The model under review builds one solid part; all positions refer to its coordinate system, in mm. A direction names the side the tool comes from. Round coordinates to 2 decimals unless told otherwise and drop trailing zeros. Write each loop counter-clockwise with the first axis right and the second up, starting at its lowest first coordinate (ties: lowest second). Pieces come first, ordered by that corner, then holes. Notation, with made-up numbers: (-39, 37) -> (-32, 37) arc R6 cw to (-32, 43) -> close; hole circle Ø4 at (-5.5, -39.75). An arc over 180 degrees is marked (long way). Use CSV: the item, a comma, the result in double quotes. Start each with the question number.
1) Take a section at B-B, the plane x = -46.5. Give the boundary of the cut face in (y, z).
2) Mouldability with a two-part tool opening along Z and no side actions: class faces 5 (the face through (4.75, 1, 52)), 6 (the face through (-40, 2, -54)), 7 (the face through (-52, 1, -4.75)) as released by +Z, released by -Z, zero draft, split by the parting line, or undercut.
3) Take a section at A-A, the plane z = 6.5. Give the boundary of the cut face in (x, y).
4) For pin 1 Ø1.5 at (y, z) = (2, -26) entering from -X; pin 2 Ø1.5 at (x, y) = (-52, 1) entering from +Z; pin 3 Ø1.5 at (y, z) = (1.5, -52) entering from -X, all flat-tipped, find the tip position at first contact; note any pin that passes through.
5) Wall thickness on probe 1 along X at (y, z) = (2.3, 48): over which ranges is the line inside the solid? List them lowest first. Write a range as [from, to].
6) Machinability: for faces 1 (the face through (50, 1, 47)), 2 (the face through (50, 1, -47)), 3 (the face through (-52, 1, -44.75)), 4 (the face through (52, 1, 4.75)), which of the approach directions +Z, -Z, +X, -X, +Y, -Y give a long, thin tool a straight path to every point of the face, cutting with its end or side? Answer none if there is none.
from build123d import *

# Parameters (mm, degrees)
SKETCH2_W           = 100
SKETCH2_H           = 100
BOSS_EXTRUDE1_DEPTH = 3
SKETCH4_W           = 9.5
SKETCH4_H           = 3
BOSS_EXTRUDE2_DEPTH = 4
SKETCH5_W           = 9.5
SKETCH5_H           = 3
BOSS_EXTRUDE3_DEPTH = 4
SKETCH6_W           = 9.5
SKETCH6_H           = 3
BOSS_EXTRUDE4_DEPTH = 4
SKETCH7_W           = 9.5
SKETCH7_H           = 3
BOSS_EXTRUDE5_DEPTH = 4


with BuildPart() as part:
    # Sketch2 → Boss-Extrude1 (new body)
    with BuildSketch(Plane(origin=(0, 0, 0), x_dir=(1, 0, 0), z_dir=(0, 1, 0))):
        Rectangle(SKETCH2_W, SKETCH2_H)
    extrude(amount=BOSS_EXTRUDE1_DEPTH)

    # Sketch4 → Boss-Extrude2 (add)
    with BuildSketch(Plane.XY.offset(50)):
        with Locations((-40, 1.5)):
            Rectangle(SKETCH4_W, SKETCH4_H)
        with Locations((-20, 1.5)):
            Rectangle(SKETCH4_W, SKETCH4_H)
        with Locations((0, 1.5)):
            Rectangle(SKETCH4_W, SKETCH4_H)
        with Locations((20, 1.5)):
            Rectangle(SKETCH4_W, SKETCH4_H)
        with Locations((40, 1.5)):
            Rectangle(SKETCH4_W, SKETCH4_H)
    extrude(amount=BOSS_EXTRUDE2_DEPTH)

    # Sketch5 → Boss-Extrude3 (add)
    with BuildSketch(Plane.ZY.offset(50)):
        with Locations((-40, 1.5)):
            Rectangle(SKETCH5_W, SKETCH5_H)
        with Locations((-20, 1.5)):
            Rectangle(SKETCH5_W, SKETCH5_H)
        with Locations((0, 1.5)):
            Rectangle(SKETCH5_W, SKETCH5_H)
        with Locations((20, 1.5)):
            Rectangle(SKETCH5_W, SKETCH5_H)
        with Locations((40, 1.5)):
            Rectangle(SKETCH5_W, SKETCH5_H)
    extrude(amount=BOSS_EXTRUDE3_DEPTH)

    # Sketch6 → Boss-Extrude4 (add)
    with BuildSketch(Plane(origin=(50, 0, 0), x_dir=(0, 0, -1), z_dir=(1, 0, 0))):
        with Locations((-40, 1.5)):
            Rectangle(SKETCH6_W, SKETCH6_H)
        with Locations((-20, 1.5)):
            Rectangle(SKETCH6_W, SKETCH6_H)
        with Locations((0, 1.5)):
            Rectangle(SKETCH6_W, SKETCH6_H)
        with Locations((20, 1.5)):
            Rectangle(SKETCH6_W, SKETCH6_H)
        with Locations((40, 1.5)):
            Rectangle(SKETCH6_W, SKETCH6_H)
    extrude(amount=BOSS_EXTRUDE4_DEPTH)

    # Sketch7 → Boss-Extrude5 (add)
    with BuildSketch(Plane(origin=(0, 0, -50), x_dir=(-1, 0, 0), z_dir=(0, 0, -1))):
        with Locations((-40, 1.5)):
            Rectangle(SKETCH7_W, SKETCH7_H)
        with Locations((-20, 1.5)):
            Rectangle(SKETCH7_W, SKETCH7_H)
        with Locations((0, 1.5)):
            Rectangle(SKETCH7_W, SKETCH7_H)
        with Locations((20, 1.5)):
            Rectangle(SKETCH7_W, SKETCH7_H)
        with Locations((40, 1.5)):
            Rectangle(SKETCH7_W, SKETCH7_H)
    extrude(amount=BOSS_EXTRUDE5_DEPTH)


solid = part.part
Values found:
1,outline,"(0, -50) -> (3, -50) -> (3, 50) -> (0, 50) -> close"
2,face 5,"zero draft"
2,face 6,"released by -Z"
2,face 7,"undercut"
3,outline,"(-50, 0) -> (50, 0) -> (50, 3) -> (-50, 3) -> close"
4,pin 1,"x = -50"
4,pin 2,"z = 44.75"
4,pin 3,"x = -44.75"
5,probe 1,"[-50, 50]"
6,face 1,"+Z, +X, +Y, -Y"
6,face 2,"-Z, +X, +Y, -Y"
6,face 3,"-Z, -X, +Y, -Y"
6,face 4,"+X, +Y, -Y"
